```python
from build123d import *

# Parameters (mm, degrees)
F0_W     = 3
F0_H     = 3
F0_H_2   = 6
F1_DEPTH = 3
F2_R     = 0.75
F3_DEPTH = 25


with BuildPart() as f1:
    # F0 (on Top) → F1 (new body)
    with BuildSketch(Plane.XY):
        with Locations((0, 3)):
            Rectangle(F0_W, F0_H)
        Rectangle(F0_W, F0_H)
        with Locations((-3, 0)):
            Rectangle(F0_W, F0_H)
        with Locations((0, -4.5)):
            Rectangle(F0_W, F0_H_2)
        with Locations((3, 0)):
            Rectangle(F0_W, F0_H)
    extrude(amount=F1_DEPTH)

    # F2 (on face) → F3 (cut)
    with BuildSketch(Plane(origin=(-1.5, 0, 0), x_dir=(0, -1, 0), z_dir=(-1, 0, 0))):
        with Locations((-3, 1.5)):
            Circle(F2_R)
    extrude(amount=-F3_DEPTH, mode=Mode.SUBTRACT)


solid = f1.part
```
Could you check a few things on this model? Use its own coordinates, in mm. A direction names the side the tool comes from. Round coordinates to 2 decimals unless told otherwise and drop trailing zeros. Loops run counter-clockwise (first coordinate to the right, second up) from the corner with the lowest first, then second, coordinate; pieces in that order, holes last. Notation, with made-up numbers: M -27,29 L -4,29 A9 cw -4,43 Z; hole C 35,-30.75 d8. An arc over 180 degrees is marked long. Write item = value, one per line.
1. Will these pins go through, and if not, where does the flat tip stop? P1, Ø0.9, axis at x = 3, z = 1, coming from the -Y side; P2, Ø2, axis at x = 3.5, y = -6, coming from the +Z side; P3, Ø1.5, axis at y = -5.5, z = 1, coming from the -X side.
Results below:
P1 = -1.5
P2 = through
P3 = -1.5
2. Which directions (+Z, -Z, +X, -X, +Y, -Y) give clear straight access to the entire face, cutting with the end or side of a thin tool? Please do faces 1 (the face through (-3, -1.5, 1)), 2 (the face through (1.5, -5, 1)), 3 (the face through (-3, 1.5, 1)).
Results below:
face_1 = +Z, -Z, -X, -Y
face_2 = +Z, -Z, +X, -Y
face_3 = +Z, -Z, -X, +Y
3. I need wall thicknesses on probe 1 along Z at (x, y) = (0.05, 3); probe 2 along X at (y, z) = (-6.25, 0.35). Which ranges of each line are inside material? Lowest first, please.
Results below:
probe_1 = 0 to 0.75, 2.25 to 3
probe_2 = -1.5 to 1.5
4. I want a section at B-B, the plane z = 1.5. Write out the boundary of the cut face in (x, y).
Results below:
outline = M -4.5,-1.5 L -1.5,-1.5 L -1.5,-7.5 L 1.5,-7.5 L 1.5,-1.5 L 4.5,-1.5 L 4.5,1.5 L 1.5,1.5 L 1.5,2.25 L -1.5,2.25 L -1.5,1.5 L -4.5,1.5 Z; M -1.5,3.75 L 1.5,3.75 L 1.5,4.5 L -1.5,4.5 Z
5. I want a section at D-D, the plane z = 0.4. Write out the boundary of the cut face in (x, y), and give its area (3 significant figures).
Results below:
outline = M -4.5,-1.5 L -1.5,-1.5 L -1.5,-7.5 L 1.5,-7.5 L 1.5,-1.5 L 4.5,-1.5 L 4.5,1.5 L 1.5,1.5 L 1.5,4.5 L -1.5,4.5 L -1.5,1.5 L -4.5,1.5 Z
area = 54.0 mm²
6. I want a section at C-C, the plane x = -1.25. Write out the boundary of the cut face in (y, z).
Results below:
outline = M -7.5,0 L 4.5,0 L 4.5,3 L -7.5,3 Z; hole C 3,1.5 d1.5
7. I want a section at A-A, the plane y = 3. Write out the boundary of the cut face in (x, z), and give its area (3 significant figures).
Results below:
outline = M -1.5,0 L 1.5,0 L 1.5,0.75 L -1.5,0.75 Z; M -1.5,2.25 L 1.5,2.25 L 1.5,3 L -1.5,3 Z
area = 4.50 mm²
8. Thinking about a two-plate mould opening in Z: for faces 4 (the face through (0, -7.5, 1)), 5 (the face through (-0.021, 3.595, 1.044)), 6 (the face through (0, -1, 3)), which applies, +Z half, -Z half, draft (parallel to the pull), parting line (faces both ways), or undercut?
Results below:
face_4 = draft
face_5 = undercut
face_6 = +Z half
